Autodesk Inventor part; units mm, degrees
ref_plane "YZ Plane" through (0, 0, 0) normal (1, 0, 0) x (0, 1, 0)
ref_plane "XZ Plane" through (0, 0, 0) normal (0, 1, 0) x (-1, 0, 0)
ref_plane "XY Plane" through (0, 0, 0) normal (0, 0, 1) x (1, 0, 0)
sketch "Sketch1" plane through (0, 0, 0) normal (0, 0, 1) x (1, 0, 0)
  line L0 (-13.1614, 0) -> (78.9686, 0)
  line L1 (0, -5.1729) -> (0, 10.0373)
  line L2 (0, 7) -> (15, 7)
  line L3 (15, 7) -> (15, 7.5)
  line L4 (15, 7.5) -> (61.6144, 7.5)
  line L5 (61.6144, 7.5) -> (61.6144, 0) construction
  line L6 (0, 5.1) -> (47.0555, 5.1)
  line L7 (47.0555, 5.1) -> (50, 0)
  arc A0 (65, 0) -> (61.6144, 7.5) centre (55, 0) ccw
  circle A1 centre (57, 0) radius 3
  line L8 (15, 7.5) -> (14.5, 7)
  point P0 (0, 0)
  dimension "d0" = 10.2
  dimension "d2" = 14
  dimension "d3" = 15
  dimension "d5" = 60
  dimension "d6" = 50
  dimension "d8" = 15
  dimension "d9" = 10
  dimension "d10" = 6
  dimension "d12" = 65
  dimension "d13" = 0.5
  dimension "d14" = 0.5
  dimension "d15" = 57
revolve "Revolution1" add sketch "Sketch1" angle 360 about axis through (-10, 0, 0) along (1, 0, 0) picked at (56.166, 1.3672) contours A1 L0 L7 L6 L1 L2 L3 L4 A0 | L0 A1 | L3 L2 L8
extrude "Extrusion1" cut sketch "Sketch1" along normal through all both and the other way through all contours A1 L0 | L0 A1
fillet "Fillet1" radius 0.5 2 edges at (54, 0.0092, 7.5) (54, 0.0092, -7.5)
equation "\"d13\" = d14"
properties part number "TW1-004"
Geometry check sheet. Reference: the model listing, model coordinates, mm. A direction names the side the tool comes from. Coordinates: 2 decimals unless noted, no trailing zeros. Write each loop counter-clockwise with the first axis right and the second up, starting at its lowest first coordinate (ties: lowest second). Pieces come first, ordered by that corner, then holes. Notation, with made-up numbers: M 27.25,46.5 L 61.25,46.5 A16 cw 61.25,60.5 Z; hole C -10.75,33.25 d7. An arc over 180 degrees is marked long. Use one line per item in the form item = value. Start each with the question number.
1) Go/stop test with flat-tipped pins: pin 1 Ø1.5 at (y, z) = (0.5, -2.5) entering from -X (3 decimals); pin 2 Ø1.5 at (x, y) = (48, -5) entering from -Z; pin 3 Ø1.5 at (y, z) = (5.5, -6) entering from +X. Record where each tip stops, or that it passes through.
2) Section check B-B on x = 46. Enter the section's corners in (y, z), and give its area (3 significant figures).
3) Release check for a two-part mould opening along Z. For faces 3 (the cylindrical face through (38.63, 6.93, -2.87)), 4 (the conical face through (49.49, 0.84, -0.27)), 5 (the cylindrical face through (23.9, 2.4, -4.5)), 6 (the cylindrical face through (58.61, -2.53, -0.1)) record: pulls with the +Z half, pulls with the -Z half, needs draft (parallel to the pull), parting line crosses it, or undercut.
4) Section check A-A on x = 4. Enter the section's corners in (y, z).
5) Set-up check for faces 1 (the cylindrical face through (7.352, 6.466, -2.681)), 2 (the flat face through (0, -5, -2)): record each of +Z, -Z, +X, -X, +Y, -Y from which the full face is reachable in a straight line by a thin tool's end or side.
6) Thickness scan on probe 1 along Z at (x, y) = (5, -2.25); probe 2 along X at (y, z) = (1.25, -1.5); probe 3 along Y at (x, z) = (57, 1.75). Record the ranges inside material, lowest first. Write a range as from..to.
Responses:
q1.pin_1 = 48.095
q1.pin_2 = -6.18
q1.pin_3 = 61.74
q2.outline = C 0,0 d15; hole C 0,0 d10.2
q2.area = 95.0 mm2
q3.face_3 = parting line crosses it
q3.face_4 = undercut
q3.face_5 = undercut
q3.face_6 = needs draft
q4.outline = C 0,0 d14; hole C 0,0 d10.2
q5.face_1 = -X
q5.face_2 = +Z, -Z, -X, +Y, -Y
q6.probe_1 = -6.63..-4.58, 4.58..6.63
q6.probe_2 = 48.87..54.27, 59.73..64.81
q6.probe_3 = -7.29..-3, 3..7.29
